```python
from build123d import *

# Parameters (mm, degrees)
F0_R      = 12.7
F1_DEPTH  = 50.8
F1_FACE_R = 12.7
F2_DEPTH  = 50.8


with BuildPart() as f1:
    # F0 (on Front) → F1 (new body)
    with BuildSketch(Plane.XZ):
        Polygon((38.1, 50.8), (0, 50.8), (0, 0), (76.2, 0), (76.2, 25.4), align=None)
        with Locations((38.1, 25.020719)):
            Circle(F0_R, mode=Mode.SUBTRACT)
    extrude(amount=-F1_DEPTH)

    # F1_face (on face) → F2 (join)
    with BuildSketch(Plane(origin=(33.833102, 0, 22.622123), x_dir=(1, 0, 0), z_dir=(0, -1, 0))):
        Polygon((4.266898, 28.177877), (-33.833102, 28.177877), (-33.833102, -22.622123), (42.366898, -22.622123), (42.366898, 2.777877), align=None)
        with Locations((4.266898, 2.398595)):
            Circle(F1_FACE_R, mode=Mode.SUBTRACT)
    extrude(amount=-F2_DEPTH)


solid = f1.part
```
Geometry check sheet. Reference: the model listing, model coordinates, mm. Round coordinates to 2 decimals unless told otherwise and drop trailing zeros. Loops run counter-clockwise (first coordinate to the right, second up) from the corner with the lowest first, then second, coordinate; pieces in that order, holes last. Notation, with made-up numbers: (-22.75, -31.75) - (10.25, -31.75) arc R25 cw to (10.25, -2.75) - close; hole circle Ø3 at (-33, 25). An arc over 180 degrees is marked (long way). Use a Markdown table: item, result.
Q1. Go/stop test with flat-tipped pins: P1, Ø8, axis at y = 23.5, z = 43.5, coming from the +X side; P2, Ø1, axis at y = 9.5, z = 37.5, coming from the +X side; P3, Ø10, axis at y = 26, z = 37.5, coming from the +X side. Record where each tip stops, or that it passes through.
Solutions:
| item | result |
|---|---|
| P1 | stops at x = 55.05 |
| P2 | stops at x = 58.8 |
| P3 | stops at x = 65.55 |
Q2. Cross-section at C-C on y = 20. Record the cut outline in (x, z), plus the area to 3 significant figures.
Solutions:
| item | result |
|---|---|
| outline | (0, 0) - (76.2, 0) - (76.2, 25.4) - (38.1, 50.8) - (0, 50.8) - close; hole (25.4, 25.02) arc R12.7 ccw to (50.8, 25.02) arc R12.7 ccw to start |
| area | 2,880 mm2 |
Q3. Cross-section at D-D on z = 47. Record the cut outline in (x, y), plus the area to 3 significant figures.
Solutions:
| item | result |
|---|---|
| outline | (0, 0) - (43.8, 0) - (43.8, 50.8) - (0, 50.8) - close |
| area | 2,230 mm2 |
Q4. Material ranges on line 1 (X direction, y = 5.5, z = 26.5); line 2 (X direction, y = 25, z = 27); line 3 (Z direction, x = 29.5, y = 7), recorded low to high.
Solutions:
| item | result |
|---|---|
| line 1 | x = 0 to 25.49, 50.71 to 74.55 |
| line 2 | x = 0 to 25.56, 50.64 to 73.8 |
| line 3 | z = 0 to 15.68, 34.37 to 50.8 |
Q5. Cross-section at B-B on x = 48. Record the cut outline in (y, z), plus the area to 3 significant figures.
Solutions:
| item | result |
|---|---|
| outline | (0, 0) - (50.8, 0) - (50.8, 17.07) - (0, 17.07) - close; (0, 32.98) - (50.8, 32.98) - (50.8, 44.2) - (0, 44.2) - close |
| area | 1,440 mm2 |
Q6. Cross-section at A-A on z = 36. Record the cut outline in (x, y), plus the area to 3 significant figures.
Solutions:
| item | result |
|---|---|
| outline | (0, 0) - (31.72, 0) - (31.72, 50.8) - (0, 50.8) - close; (44.48, 0) - (60.3, 0) - (60.3, 50.8) - (44.48, 50.8) - close |
| area | 2,410 mm2 |
